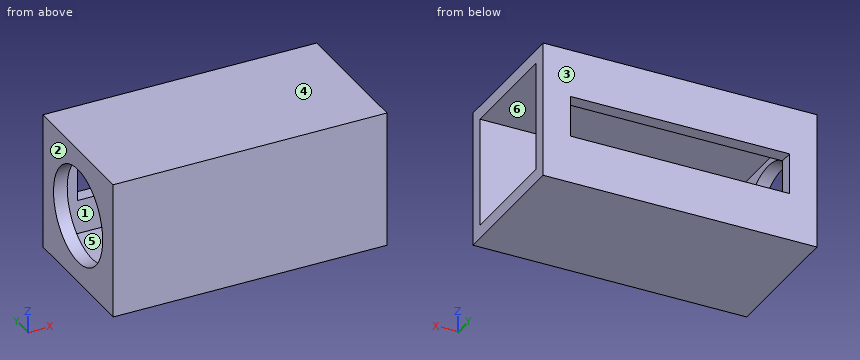
```python
from build123d import *

# Parameters (mm, degrees)
SKETCH1_W           = 20
SKETCH1_H           = 10
BOSS_EXTRUDE1_DEPTH = 10
SHELL1_T            = -1
CUT_EXTRUDE1_REACH  = 22
SKETCH3_R           = 3.5
CUT_EXTRUDE2_REACH  = 12
SKETCH5_W           = 16
SKETCH5_H           = 3


with BuildPart() as part:
    # Sketch1 → Boss-Extrude1 (new body)
    with BuildSketch(Plane.XY):
        Rectangle(SKETCH1_W, SKETCH1_H)
    extrude(amount=BOSS_EXTRUDE1_DEPTH)

    # Shell1
    shell1_openings = [part.faces().sort_by_distance(p)[0] for p in [
        (10, 0, 5),
    ]]
    offset(amount=SHELL1_T, openings=shell1_openings, kind=Kind.INTERSECTION)

    # Sketch3 → Cut-Extrude1 (cut, up to next)
    with BuildSketch(Plane.ZY.offset(10), mode=Mode.PRIVATE) as cut_extrude1_sk1:
        with Locations((5, 0)):
            Circle(SKETCH3_R)
    cut_extrude1_tool1 = extrude(cut_extrude1_sk1.sketch, amount=-CUT_EXTRUDE1_REACH, mode=Mode.PRIVATE) & part.part
    add(cut_extrude1_tool1.solids().sort_by_distance((-10, 0, 5))[0], mode=Mode.SUBTRACT)

    # Sketch5 → Cut-Extrude2 (cut, up to next)
    with BuildSketch(Plane(origin=(0, 5, 0), x_dir=(1, 0, 0), z_dir=(0, 1, 0)), mode=Mode.PRIVATE) as cut_extrude2_sk1:
        with Locations((0, -5)):
            Rectangle(SKETCH5_W, SKETCH5_H)
    cut_extrude2_tool1 = extrude(cut_extrude2_sk1.sketch, amount=-CUT_EXTRUDE2_REACH, mode=Mode.PRIVATE) & part.part
    add(cut_extrude2_tool1.solids().sort_by_distance((0, 5, 5))[0], mode=Mode.SUBTRACT)


solid = part.part
```
Design review of the part built by this model. Coordinates are the model's own, in mm. Face numbers are marked on the shaded views. A direction names the side the tool comes from. Coordinates: 2 decimals unless noted, no trailing zeros. Loops run counter-clockwise (first coordinate to the right, second up) from the corner with the lowest first, then second, coordinate; pieces in that order, holes last. Notation, with made-up numbers: (-19.5, 25) -> (36.5, 25) arc R20 cw to (36.5, 62) -> close; hole circle Ø6 at (17, 74). An arc over 180 degrees is marked (long way). Answer as a JSON object with one key per item and string values.
Q1. The part is to be moulded in two halves that separate along Z. For the marked faces 3, 4, 5 and 6, say which applies: +Z half, -Z half, draft (parallel to the pull), parting line (faces both ways), or undercut.
Answer block:
{"face 3": "draft", "face 4": "+Z half", "face 5": "undercut", "face 6": "undercut"}
Q2. To check wall thickness, follow L1, parallel to Y at x = -9.25, z = 5; L2, parallel to Z at x = 7.5, y = 1; L3, parallel to Y at x = -0.75, z = 7.5. State the ranges of each line that lie inside material, in increasing order.
Answer block:
{"L1": "y = -5 to -3.5, 3.5 to 5", "L2": "z = 0 to 1, 9 to 10", "L3": "y = -5 to -4, 4 to 5"}
Q3. Take a section at B-B on z = 5. Give the boundary of the cut face in (x, y).
Answer block:
{"outline": "(-10, -5) -> (10, -5) -> (10, -4) -> (-9, -4) -> (-9, -3.5) -> (-10, -3.5) -> close; (-10, 3.5) -> (-9, 3.5) -> (-9, 4) -> (-8, 4) -> (-8, 5) -> (-10, 5) -> close; (8, 4) -> (10, 4) -> (10, 5) -> (8, 5) -> close"}
Q4. Take a section at C-C on z = 7. Give the boundary of the cut face in (x, y).
Answer block:
{"outline": "(-10, -5) -> (10, -5) -> (10, -4) -> (-9, -4) -> (-9, -2.87) -> (-10, -2.87) -> close; (-10, 2.87) -> (-9, 2.87) -> (-9, 4) -> (10, 4) -> (10, 5) -> (-10, 5) -> close"}
Q5. Tool access review of the marked faces 1 and 2: name each direction out of +Z, -Z, +X, -X, +Y, -Y from which nothing blocks a thin tool from reaching the whole face with its end or side.
Answer block:
{"face 1": "+X", "face 2": "+Z, -Z, -X, +Y, -Y"}
Q6. Take a section at A-A on y = 0. Give the boundary of the cut face in (x, z), plus the area to 3 significant figures.
Answer block:
{"outline": "(-10, 0) -> (10, 0) -> (10, 1) -> (-9, 1) -> (-9, 1.5) -> (-10, 1.5) -> close; (-10, 8.5) -> (-9, 8.5) -> (-9, 9) -> (10, 9) -> (10, 10) -> (-10, 10) -> close", "area": "41.0 mm^2"}
Q7. Take a section at D-D on z = 3.75. Give the boundary of the cut face in (x, y).
Answer block:
{"outline": "(-10, -5) -> (10, -5) -> (10, -4) -> (-9, -4) -> (-9, -3.27) -> (-10, -3.27) -> close; (-10, 3.27) -> (-9, 3.27) -> (-9, 4) -> (-8, 4) -> (-8, 5) -> (-10, 5) -> close; (8, 4) -> (10, 4) -> (10, 5) -> (8, 5) -> close"}
